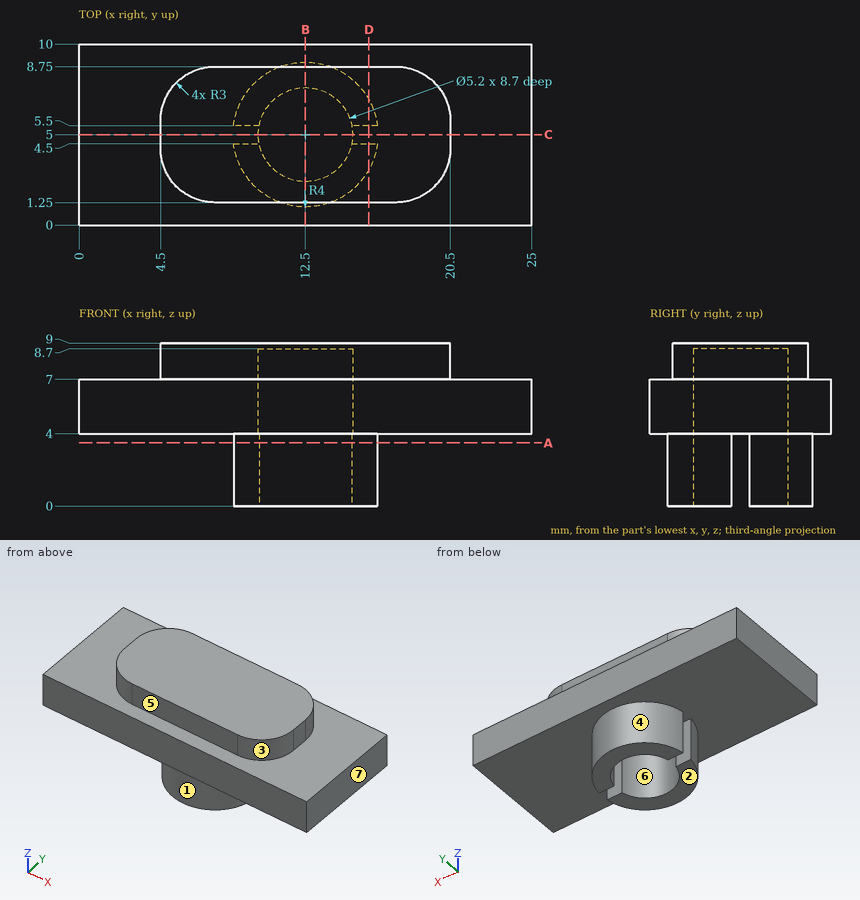
Answer from the drawing. Dimensions are ordinates in mm from the lowest x, y and z of the part. A direction names the side the tool comes from. Round coordinates to 2 decimals unless told otherwise and drop trailing zeros. Write each loop counter-clockwise with the first axis right and the second up, starting at its lowest first coordinate (ties: lowest second). Pieces come first, ordered by that corner, then holes. Notation, with made-up numbers: (-34, -38.5) -> (-25, -38.5) arc R5 ccw to (-25, -31.5) -> close; hole circle Ø7 at (87, 4). An arc over 180 degrees is marked (long way). Answer in a Markdown table with one row per item. Add a question column.
1) Given P1, Ø0.7, axis at x = 9, z = 2.5, coming from the -Y side; P2, Ø4, axis at x = 4.5, z = 1.5, coming from the +Y side; P3, Ø1.6, axis at x = 15.5, z = 2, coming from the -Y side; P4, Ø0.7, axis at x = 9, z = 1.5, coming from the +Y side, each flat-ended and moving along its own axis, determine where each tip first touches the part or whether it passes through.
2) Which of the six approach directions +Z, -Z, +X, -X, +Y, -Y give full straight-line access (tool end or side, diameter ignored) to the marked faces 1, 2, 3 and 4?
3) Find section C-C, the plane y = 5. Determine the outline of the cut face in (x, z).
4) Consider line 1 (Y direction, x = 12.5, z = 4.5); line 2 (X direction, y = 5, z = 4.75); line 3 (Z direction, x = 7.25, y = 9.25). Determine where each line is inside the solid, lowest interval first.
5) Determine the mould class of the marked faces 5, 6 and 7 for opening direction Y: pulls with the +Y half, pulls with the -Y half, needs draft (parallel to the pull), parting line crosses it, or undercut.
6) Find section D-D, the plane x = 16. Determine the outline of the cut face in (y, z), and give its area (3 significant figures).
7) Find section B-B, the plane x = 12.5. Determine the outline of the cut face in (y, z), and give its area (3 significant figures).
8) Find section A-A, the plane z = 3.5. Determine the outline of the cut face in (x, y), and give its area (3 significant figures).
Findings below:
| question | item | result |
|---|---|---|
| 1 | P1 | y = 2.53 |
| 1 | P2 | through |
| 1 | P3 | y = 1.66 |
| 1 | P4 | y = 7.47 |
| 2 | face 1 | -Z, -Y |
| 2 | face 2 | -Z, +X, -X, +Y, -Y |
| 2 | face 3 | +Z, +X, -Y |
| 2 | face 4 | -Z, +Y |
| 3 | outline | (0, 4) -> (9.9, 4) -> (9.9, 8.7) -> (15.1, 8.7) -> (15.1, 4) -> (25, 4) -> (25, 7) -> (20.5, 7) -> (20.5, 9) -> (4.5, 9) -> (4.5, 7) -> (0, 7) -> close |
| 4 | line 1 | 0 to 2.4, 7.6 to 10 |
| 4 | line 2 | 0 to 9.9, 15.1 to 25 |
| 4 | line 3 | 4 to 7 |
| 5 | face 5 | pulls with the -Y half |
| 5 | face 6 | undercut |
| 5 | face 7 | needs draft |
| 6 | outline | (0, 4) -> (3.06, 4) -> (3.06, 0) -> (4.5, 0) -> (4.5, 4) -> (5.5, 4) -> (5.5, 0) -> (6.94, 0) -> (6.94, 4) -> (10, 4) -> (10, 7) -> (8.75, 7) -> (8.75, 9) -> (1.25, 9) -> (1.25, 7) -> (0, 7) -> close |
| 6 | area | 56.5 mm² |
| 7 | outline | (0, 4) -> (1, 4) -> (1, 0) -> (2.4, 0) -> (2.4, 8.7) -> (7.6, 8.7) -> (7.6, 0) -> (9, 0) -> (9, 4) -> (10, 4) -> (10, 7) -> (8.75, 7) -> (8.75, 9) -> (1.25, 9) -> (1.25, 7) -> (0, 7) -> close |
| 7 | area | 31.8 mm² |
| 8 | outline | (8.53, 4.5) arc R4 ccw to (16.47, 4.5) -> (15.05, 4.5) arc R2.6 cw to (9.95, 4.5) -> close; (8.53, 5.5) -> (9.95, 5.5) arc R2.6 cw to (15.05, 5.5) -> (16.47, 5.5) arc R4 ccw to start |
| 8 | area | 26.2 mm² |
